The model under review builds one solid part; all positions refer to its coordinate system, in mm. Face numbers are marked on the shaded views. A direction names the side the tool comes from. Coordinates: 2 decimals unless noted, no trailing zeros. Write each loop counter-clockwise with the first axis right and the second up, starting at its lowest first coordinate (ties: lowest second). Pieces come first, ordered by that corner, then holes. Notation, with made-up numbers: (74.25, -36.75) - (120.25, -36.75) arc R15 cw to (120.25, -22.75) - close; hole circle Ø3 at (60, 32.5). An arc over 180 degrees is marked (long way). Put each result on its own line as item: value.
Autodesk Fusion 360 part; units mm, degrees
sketch "Sketch1" plane through (0, 0, 0) normal (0, 1, 0) x (1, 0, 0)
  line L0 (0, 0) -> (16, 0)
  line L1 (16, 0) -> (16, 12)
  line L2 (16, 12) -> (7.5, 12)
  line L3 (7.5, 6) -> (0, 6)
  line L4 (7.5, 12) -> (7.5, 10)
  line L5 (7.5, 10) -> (7, 10)
  line L6 (6.5, 9.5) -> (6.5, 9.5)
  line L7 (7, 9) -> (7.5, 9)
  line L8 (7.5, 9) -> (7.5, 6)
  arc A0 (6.5, 9.5) -> (7, 9) centre (7, 9.5) ccw
  arc A1 (7, 10) -> (6.5, 9.5) centre (7, 9.5) ccw
  line L9 (-7, 9) -> (-7.5, 9)
  line L10 (-7.5, 10) -> (-7, 10)
  arc A2 (-6.5, 9.5) -> (-7, 10) centre (-7, 9.5) ccw
  arc A3 (-7, 9) -> (-6.5, 9.5) centre (-7, 9.5) ccw
  line L11 (-16, 12) -> (-7.5, 12)
  line L12 (-16, 0) -> (-16, 12)
  line L13 (-6.5, 9.5) -> (-6.5, 9.5)
  line L14 (0, 0) -> (-16, 0)
  line L15 (-7.5, 6) -> (0, 6)
  line L16 (-7.5, 12) -> (-7.5, 10)
  line L17 (-7.5, 9) -> (-7.5, 6)
  point P0 (6.5, 10)
  point P1 (6.5, 9)
  point P2 (-6.5, 9)
  point P3 (-6.5, 10)
  dimension "d1" = 16
  dimension "d2" = 12
  dimension "d3" = 8.5
  dimension "d4" = 6
  dimension "d5" = 7.5
  dimension "d6" = 1
  dimension "d7" = 1
  dimension "d8" = 1
  dimension "d9" = 0.5
  dimension "d10" = 0.5
extrude "Extrude1" add sketch "Sketch1" along normal blind 58.8
sketch "Sketch2" plane through (0, 0, 0) normal (0, 0, 1) x (-1, 0, 0)
  line L0 (16, 0) -> (-16, 0)
  line L1 (-16, 0) -> (-16, -58.8)
  line L2 (-16, -58.8) -> (16, -58.8)
  line L3 (16, -58.8) -> (16, 0)
  line L4 (0, -29.4) -> (-12.5, -29.4)
  line L5 (-12.5, -29.4) -> (-12.5, -41.9)
  line L6 (-12.5, -41.9) -> (0, -41.9)
  line L7 (0, -41.9) -> (0, -29.4)
  circle A0 centre (-12.5, -41.9) radius 1.5
  circle A1 centre (12.5, -41.9) radius 1.5
  circle A2 centre (12.5, -16.9) radius 1.5
  circle A3 centre (-12.5, -16.9) radius 1.5
  dimension "d13" = 12.5
  dimension "d14" = 12.5
  dimension "d15" = 3
extrude "Extrude2" cut sketch "Sketch2" against normal blind 6 contours L5 L6 A0 | L5 L6 A0 | A1 | A2 | A3
chamfer "Chamfer1" distance 1 angle 45 4 edges at (-16, 29.4, 0) (-16, 29.4, -12) (16, 29.4, 0) (16, 29.4, -12)
chamfer "Chamfer2" distance 0.2 angle 45 4 edges at (-11.1015, 41.3576, 0) (13.8985, 41.3576, 0) (13.8985, 16.3576, 0) (-11.1015, 16.3576, 0)
sketch "Sketch3" plane through (0, 0, 0) normal (0, -1, 0) x (1, 0, 0)
  line L0 (15, -12) -> (16, -11)
  line L1 (16, -11) -> (16, -1)
  line L2 (16, -1) -> (15, 0)
  line L3 (15, 0) -> (-15, 0)
  line L4 (-15, 0) -> (-16, -1)
  line L5 (-16, -1) -> (-16, -11)
  line L6 (-16, -11) -> (-15, -12)
  line L7 (-15, -12) -> (-7.5, -12)
  line L8 (-7.5, -12) -> (-7.5, -10)
  line L9 (-7.5, -10) -> (-7, -10)
  arc A0 (-7, -10) -> (-7, -9) centre (-7, -9.5) ccw
  line L10 (-7, -9) -> (-7.5, -9)
  line L11 (-7.5, -9) -> (-7.5, -6)
  line L12 (-7.5, -6) -> (7.5, -6)
  line L13 (7.5, -6) -> (7.5, -9)
  line L14 (7.5, -9) -> (7, -9)
  arc A1 (7, -9) -> (7, -10) centre (7, -9.5) ccw
  line L15 (7, -10) -> (7.5, -10)
  line L16 (7.5, -10) -> (7.5, -12)
  line L17 (7.5, -12) -> (15, -12)
  circle A2 centre (-10, -3.0186) radius 2.5
  circle A3 centre (10, -3.0186) radius 2.5
  dimension "d22" = 5
extrude "Extrude3" add sketch "Sketch3" along normal blind 4.5 contours A2 | A3
chamfer "Chamfer3" distance 0.5 angle 45 2 edges at (-12.3308, -4.5, -3.9226) (7.6692, -4.5, -3.9226)
sketch "Sketch4" plane through (0, -4.5, 0) normal (0, -1, 0) x (1, 0, 0)
  circle A0 centre (-10, -3.0186) radius 2
  line L0 (-11.0354, -2.0354) -> (-10.9646, -1.9646)
  line L1 (-9.0012, -1.9676) -> (-8.9312, -2.039)
  line L2 (-11.035, -3.9643) -> (-10.965, -4.0357)
  line L3 (-9.0354, -4.0354) -> (-8.9646, -3.9646)
  line L4 (-11.0337, -3.8229) -> (-10.2039, -3.0082)
  line L5 (-9.9898, -2.7981) -> (-9.1426, -1.9663)
  line L6 (-10.8232, -1.9646) -> (-9.9898, -2.7981)
  line L7 (-9.7777, -3.0102) -> (-8.9646, -3.8232)
  line L8 (-10.8236, -4.037) -> (-9.9918, -3.2204)
  line L9 (-9.7777, -3.0102) -> (-8.9325, -2.1804)
  line L10 (-11.0354, -2.1768) -> (-10.2039, -3.0082)
  line L11 (-9.9918, -3.2204) -> (-9.1768, -4.0354)
  arc A1 (-11.0354, -2.0354) -> (-11.0354, -2.1768) centre (-10.9646, -2.1061) ccw
  arc A2 (-10.8232, -1.9646) -> (-10.9646, -1.9646) centre (-10.8939, -2.0354) ccw
  arc A3 (-9.0012, -1.9676) -> (-9.1426, -1.9663) centre (-9.0726, -2.0377) ccw
  arc A4 (-8.9325, -2.1804) -> (-8.9312, -2.039) centre (-9.0025, -2.109) ccw
  arc A5 (-8.9646, -3.9646) -> (-8.9646, -3.8232) centre (-9.0354, -3.8939) ccw
  arc A6 (-9.1768, -4.0354) -> (-9.0354, -4.0354) centre (-9.1061, -3.9646) ccw
  arc A7 (-10.965, -4.0357) -> (-10.8236, -4.037) centre (-10.8936, -3.9656) ccw
  arc A8 (-11.0337, -3.8229) -> (-11.035, -3.9643) centre (-10.9637, -3.8943) ccw
  arc A9 (11.0354, -2.1768) -> (11.0354, -2.0354) centre (10.9646, -2.1061) ccw
  line L12 (11.035, -3.9643) -> (10.965, -4.0357)
  line L13 (9.7777, -3.0102) -> (8.9325, -2.1804)
  line L14 (11.0354, -2.0354) -> (10.9646, -1.9646)
  line L15 (9.9898, -2.7981) -> (9.1426, -1.9663)
  arc A10 (8.9646, -3.8232) -> (8.9646, -3.9646) centre (9.0354, -3.8939) ccw
  arc A11 (8.9312, -2.039) -> (8.9325, -2.1804) centre (9.0025, -2.109) ccw
  line L16 (9.9918, -3.2204) -> (9.1768, -4.0354)
  arc A12 (10.8236, -4.037) -> (10.965, -4.0357) centre (10.8936, -3.9656) ccw
  arc A13 (9.0354, -4.0354) -> (9.1768, -4.0354) centre (9.1061, -3.9646) ccw
  arc A14 (11.035, -3.9643) -> (11.0337, -3.8229) centre (10.9637, -3.8943) ccw
  line L17 (10.8236, -4.037) -> (9.9918, -3.2204)
  arc A15 (9.1426, -1.9663) -> (9.0012, -1.9676) centre (9.0726, -2.0377) ccw
  line L18 (10.8232, -1.9646) -> (9.9898, -2.7981)
  arc A16 (10.9646, -1.9646) -> (10.8232, -1.9646) centre (10.8939, -2.0354) ccw
  line L19 (11.0354, -2.1768) -> (10.2039, -3.0082)
  line L20 (9.0012, -1.9676) -> (8.9312, -2.039)
  line L21 (11.0337, -3.8229) -> (10.2039, -3.0082)
  line L22 (9.7777, -3.0102) -> (8.9646, -3.8232)
  line L23 (9.0354, -4.0354) -> (8.9646, -3.9646)
  point P0 (10, -3.0186)
  dimension "d30" = 0.1
  dimension "d31" = 0.1
extrude "Extrude4" cut sketch "Sketch4" against normal blind 1 contours L0 L1 L2 L3 L4 L5 L6 L7 L8 L9 L10 L11 A1 A2 A3 A4 A5 A6 A7 A8 | A9 L12 L13 L14 L15 A10 A11 L16 A12 A13 A14 L17 A15 L18 A16 L19 L20 L21 L22 L23
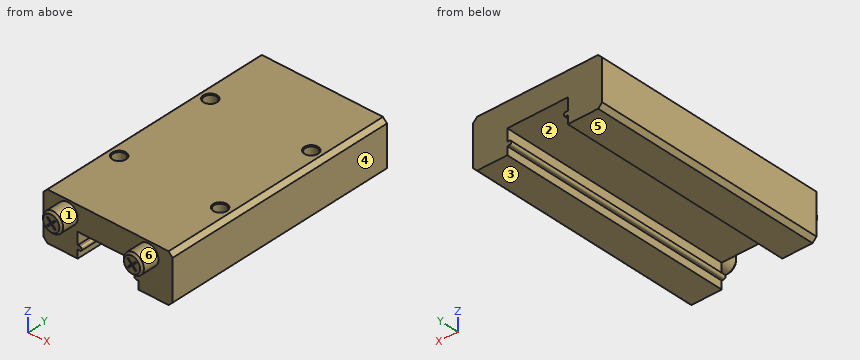
1. The part is to be moulded in two halves that separate along X. For the marked faces 4, 5 and 6, say which applies: +X half, -X half, draft (parallel to the pull), parting line (faces both ways), or undercut.
Determined:
face 4: +X half
face 5: draft
face 6: undercut
2. Consider section A-A on z = -7.75. State the section outline as (x, y) points.
Determined:
outline: (-16, 0) - (-7.5, 0) - (-7.5, 58.8) - (-16, 58.8) - close; (7.5, 0) - (16, 0) - (16, 58.8) - (7.5, 58.8) - close
3. Consider section B-B on y = 13.5. State the section outline as (x, z) points, plus the area to 3 significant figures.
Determined:
outline: (-16, -11) - (-15, -12) - (-7.5, -12) - (-7.5, -10) - (-7, -10) arc R0.5 ccw to (-7, -9) - (-7.5, -9) - (-7.5, -6) - (7.5, -6) - (7.5, -9) - (7, -9) arc R0.5 ccw to (7, -10) - (7.5, -10) - (7.5, -12) - (15, -12) - (16, -11) - (16, -1) - (15, 0) - (-15, 0) - (-16, -1) - close
area: 294 mm^2
4. To check wall thickness, follow probe 1 along X at (y, z) = (41.9, -1.65); probe 2 along Y at (x, z) = (12.5, -1.8); probe 3 along X at (y, z) = (38, -8). State the ranges of each line that lie inside material, in increasing order.
Determined:
probe 1: x = -16 to -14, -11 to 11, 14 to 16
probe 2: y = 0 to 15.4, 18.4 to 40.4, 43.4 to 58.8
probe 3: x = -16 to -7.5, 7.5 to 16
5. Machinability: for the marked faces 1, 2 and 3, which of the approach directions +Z, -Z, +X, -X, +Y, -Y give a long, thin tool a straight path to every point of the face, cutting with its end or side? Answer none if there is none.
Determined:
face 1: -Y
face 2: +Y, -Y
face 3: -Z, +X, -X, +Y, -Y
6. For pin 1 Ø2.5 at (x, y) = (12.5, 41.5) entering from +Z; pin 2 Ø6 at (x, z) = (-2.5, -8) entering from -Y; pin 3 Ø0.6 at (x, y) = (7, 35.5) entering from -Z, all flat-tipped, find the tip position at first contact; note any pin that passes through.
Determined:
pin 1: stops at z = -0.05
pin 2: stops at y = 0
pin 3: stops at z = -10
7. Consider section C-C on x = -5. State the section outline as (y, z) points, plus the area to 3 significant figures.
Determined:
outline: (0, -6) - (58.8, -6) - (58.8, 0) - (0, 0) - close
area: 353 mm^2
